from build123d import *

# Parameters (mm, degrees)
SKETCH1_R          = 22
SKETCH1_R_2        = 12.5
BASE_EXTRUDE_DEPTH = 4
IDCHAMFER_SIZE     = 2
ODCHAMFER_SIZE     = 1


with BuildPart() as part:
    # Sketch1 → Base-Extrude (new body)
    with BuildSketch(Plane(origin=(0, 0, 0), x_dir=(0, 0, -1), z_dir=(1, 0, 0))):
        Circle(SKETCH1_R)
        Circle(SKETCH1_R_2, mode=Mode.SUBTRACT)
    extrude(amount=BASE_EXTRUDE_DEPTH)

    # IDchamfer
    idchamfer_edges = [part.edges().sort_by_distance(p)[0] for p in [
        (4, 0, 12.5),
    ]]
    chamfer(idchamfer_edges, length=IDCHAMFER_SIZE)

    # ODchamfer
    odchamfer_edges = [part.edges().sort_by_distance(p)[0] for p in [
        (4, 0, 22),
    ]]
    chamfer(odchamfer_edges, length=ODCHAMFER_SIZE)


solid = part.part
The model under review builds one solid part; all positions refer to its coordinate system, in mm. Give positions to 0.01 mm unless a question says otherwise; leave off trailing zeros. Order: outer loops, then holes, each group sorted by start corner. A loop starts at its lowest first (then second) coordinate and runs counter-clockwise, first axis right, second up. Notation, with made-up numbers: M -7.5,0 L 48.5,0 A22 cw 48.5,37 Z; hole C 48.5,33 d6. An arc over 180 degrees is marked long. One line per question, with ' | ' between items. Start each with the question number.
1) Consider section A-A, the plane y = 0. Give the boundary of the cut face in (x, z), then the cut area to 3 significant figures.
2) Consider section C-C, the plane x = 1.25. Give the boundary of the cut face in (y, z), then the cut area to 3 significant figures.
3) Wall thickness on L1, parallel to Y at x = 0.7, z = 0; L2, parallel to Y at x = 2.7, z = -2.5; L3, parallel to Z at x = 2.9, y = 1.5: over which ranges is each line inside the solid? List them lowest first. Write a range as from..to.
4) Mouldability with a two-part tool opening along Y and no side actions: class faces 1 (the face through (1.479, -21.477, 4.769)), 2 (the face through (0.986, 3.755, -11.923)), 3 (the face through (0, -9, -9)) as pulls with the +Y half, pulls with the -Y half, needs draft (parallel to the pull), parting line crosses it, or undercut.
5) Clearance check with a flat-ended pin moving along its axis: P1, Ø12, axis at y = 16, z = 15, coming from the +X side. State where the tip first meets the part, or that it passes through.
Found:
1) outline: M 0,-22 L 3,-22 L 4,-21 L 4,-14.5 L 2,-12.5 L 0,-12.5 Z; M 0,12.5 L 2,12.5 L 4,14.5 L 4,21 L 3,22 L 0,22 Z | area: 71.0 mm²
2) outline: C 0,0 d44; hole C 0,0 d25 | area: 1,030 mm²
3) L1: y = -22..-12.5, 12.5..22 | L2: y = -21.86..-12.96, 12.96..21.86 | L3: z = -21.95..-13.32, 13.32..21.95
4) face 1: parting line crosses it | face 2: undercut | face 3: needs draft
5) P1: stops at x = 4
